Work out the finished part from the listing and answer in its coordinate system (mm). Give positions to 0.01 mm unless a question says otherwise; leave off trailing zeros. Order: outer loops, then holes, each group sorted by start corner. A loop starts at its lowest first (then second) coordinate and runs counter-clockwise, first axis right, second up. Notation, with made-up numbers: (63.25, 10.25) - (74.25, 10.25) arc R29 cw to (74.25, 37.25) - close; hole circle Ø8 at (-38.5, -34.5). An arc over 180 degrees is marked (long way). Write each question's results on one line, items separated by ' | '.
from build123d import *

# Parameters (mm, degrees)
SKICA1_W                 = 67
SKICA1_H                 = 107
P_IDAT_VYSUNUT_M1_DEPTH  = 3.5
ZAOBLIT1_R               = 3
SKICA2_R                 = 1.25
SKICA2_R_2               = 3
SKICA2_R_3               = 5.2
SKICA2_W                 = 41
SKICA2_H                 = 38
SKICA2_W_2               = 5.5
SKICA2_H_2               = 9
SKICA2_W_3               = 12.8
SKICA2_H_3               = 12.8
SKICA2_W_4               = 22.5
SKICA2_H_4               = 3.2
ODEBRAT_VYSUNUT_M1_DEPTH = 4.5
ZAOBLIT2_R               = 3
SKICA3_W                 = 22
SKICA3_H                 = 3
ODEBRAT_VYSUNUT_M2_DEPTH = 2
ZKOSEN_1_SIZE            = 1.3
SKICA4_W                 = 20.5
SKICA4_H                 = 8.5
ODEBRAT_VYSUNUT_M3_DEPTH = 1.2
SKICA5_W                 = 18.5
SKICA5_H                 = 6.5
ODEBRAT_VYSUNUT_M4_DEPTH = 3.3


with BuildPart() as part:
    # Skica1 → Přidat vysunutím1 (new body)
    with BuildSketch(Plane.XY):
        with Locations((33.5, 53.5)):
            Rectangle(SKICA1_W, SKICA1_H)
    extrude(amount=P_IDAT_VYSUNUT_M1_DEPTH)

    # Zaoblit1
    zaoblit1_edges = [part.edges().sort_by_distance(p)[0] for p in [
        (0, 107, 1.75),
        (67, 107, 1.75),
        (67, 0, 1.75),
        (0, 0, 1.75),
    ]]
    fillet(zaoblit1_edges, radius=ZAOBLIT1_R)

    # Skica2 → Odebrat vysunutím1 (cut, through all)
    with BuildSketch(Plane.XY.offset(3.5)):
        with Locations((6.5, 100.5)):
            Circle(SKICA2_R)
        with Locations((60.5, 100.5)):
            Circle(SKICA2_R)
        with Locations((6.5, 6.5)):
            Circle(SKICA2_R)
        with Locations((60.5, 6.5)):
            Circle(SKICA2_R)
        with Locations((7.3, 75.5)):
            Circle(SKICA2_R_2)
        with Locations((12.5, 12.5)):
            Circle(SKICA2_R_3)
        with Locations((26.5, 12.5)):
            Circle(SKICA2_R_3)
        with Locations((40.5, 12.5)):
            Circle(SKICA2_R_3)
        with Locations((54.5, 12.5)):
            Circle(SKICA2_R_3)
        with Locations((7.3, 84.5)):
            Circle(SKICA2_R_2)
        with Locations((33, 80.5)):
            Rectangle(SKICA2_W, SKICA2_H)
        with Locations((59.75, 76.5)):
            Rectangle(SKICA2_W_2, SKICA2_H_2)
        with Locations((54.5, 53.5)):
            Rectangle(SKICA2_W_3, SKICA2_H_3)
        with Locations((40.5, 53.5)):
            Rectangle(SKICA2_W_3, SKICA2_H_3)
        with Locations((26.5, 53.5)):
            Rectangle(SKICA2_W_3, SKICA2_H_3)
        with Locations((12.5, 53.5)):
            Rectangle(SKICA2_W_3, SKICA2_H_3)
        with Locations((50.65, 39.7)):
            Rectangle(SKICA2_W_4, SKICA2_H_4)
    extrude(amount=-ODEBRAT_VYSUNUT_M1_DEPTH, mode=Mode.SUBTRACT)

    # Zaoblit2
    zaoblit2_edges = [part.edges().sort_by_distance(p)[0] for p in [
        (6.1, 47.1, 1.75),
        (6.1, 59.9, 1.75),
        (18.9, 59.9, 1.75),
        (18.9, 47.1, 1.75),
        (20.1, 47.1, 1.75),
        (20.1, 59.9, 1.75),
        (32.9, 59.9, 1.75),
        (32.9, 47.1, 1.75),
        (34.1, 47.1, 1.75),
        (34.1, 59.9, 1.75),
        (46.9, 59.9, 1.75),
        (46.9, 47.1, 1.75),
        (48.1, 47.1, 1.75),
        (48.1, 59.9, 1.75),
        (60.9, 59.9, 1.75),
        (60.9, 47.1, 1.75),
    ]]
    fillet(zaoblit2_edges, radius=ZAOBLIT2_R)

    # Skica3 → Odebrat vysunutím2 (cut)
    with BuildSketch(Plane(origin=(0, 0, 0), x_dir=(-1, 0, 0), z_dir=(0, 0, -1))):
        with Locations((-33, 101)):
            Rectangle(SKICA3_W, SKICA3_H)
    extrude(amount=-ODEBRAT_VYSUNUT_M2_DEPTH, mode=Mode.SUBTRACT)

    # Zkosení1
    zkosen_1_edges = [part.edges().sort_by_distance(p)[0] for p in [
        (5.25, 6.5, 3.5),
        (59.25, 6.5, 3.5),
        (5.25, 100.5, 3.5),
        (59.25, 100.5, 3.5),
    ]]
    chamfer(zkosen_1_edges, length=ZKOSEN_1_SIZE)

    # Skica4 → Odebrat vysunutím3 (cut)
    with BuildSketch(Plane.XY.offset(3.5)):
        with Locations((16.35, 37.05)):
            Rectangle(SKICA4_W, SKICA4_H)
    extrude(amount=-ODEBRAT_VYSUNUT_M3_DEPTH, mode=Mode.SUBTRACT)

    # Skica5 → Odebrat vysunutím4 (cut, through all)
    with BuildSketch(Plane.XY.offset(2.3)):
        with Locations((16.35, 37.05)):
            Rectangle(SKICA5_W, SKICA5_H)
    extrude(amount=-ODEBRAT_VYSUNUT_M4_DEPTH, mode=Mode.SUBTRACT)


solid = part.part
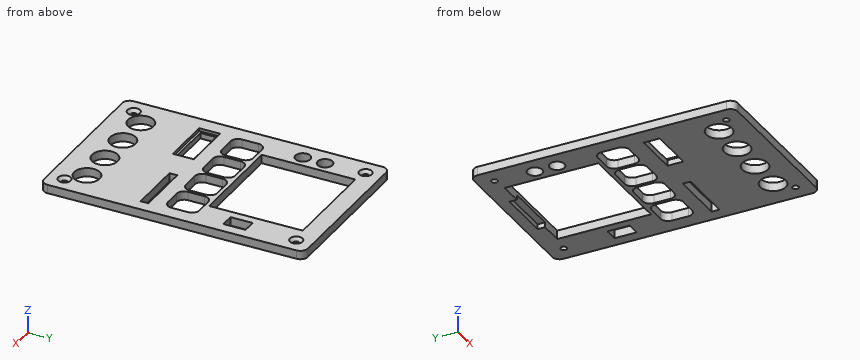
1. A cutting plane is placed at C-C, the plane z = 2.9. State how many separate pieces and enclosed holes the cut face has, then the cut area to 3 significant figures.
Answer list:
separate pieces: 1 | enclosed holes: 18 | area: 4,240 mm^2
2. A cutting plane is placed at A-A, the plane y = 12.5. Write down the section's boundary in (x, z), then the cut area to 3 significant figures.
Answer list:
outline: (0, 0) - (7.3, 0) - (7.3, 3.5) - (0, 3.5) - close; (17.7, 0) - (21.3, 0) - (21.3, 3.5) - (17.7, 3.5) - close; (31.7, 0) - (35.3, 0) - (35.3, 3.5) - (31.7, 3.5) - close; (45.7, 0) - (49.3, 0) - (49.3, 3.5) - (45.7, 3.5) - close; (59.7, 0) - (67, 0) - (67, 3.5) - (59.7, 3.5) - close | area: 88.9 mm^2
3. Given P1, Ø1.5, axis at x = 37, y = 101, coming from the -Z side, flat-ended and moving along its own axis, determine where the tip first touches the part or whether it passes through.
Answer list:
P1: z = 2
4. Straight lines are drawn through the part: line 1 (X direction, y = 53, z = 1.4); line 2 (Y direction, x = 54.5, z = 1.95); line 3 (X direction, y = 100.5, z = 0.95). For each, find the intervals that lie inside material, in ascending order. Write a range as [from, to].
Answer list:
line 1: [0, 6.1], [18.9, 20.1], [32.9, 34.1], [46.9, 48.1], [60.9, 67] | line 2: [0, 7.3], [17.7, 38.1], [41.3, 47.1], [59.9, 107] | line 3: [0, 5.25], [7.75, 22], [44, 59.25], [61.75, 67]
5. A cutting plane is placed at B-B, the plane y = 84.5. Write down the section's boundary in (x, z), then the cut area to 3 significant figures.
Answer list:
outline: (0, 0) - (4.3, 0) - (4.3, 3.5) - (0, 3.5) - close; (10.3, 0) - (12.5, 0) - (12.5, 3.5) - (10.3, 3.5) - close; (53.5, 0) - (67, 0) - (67, 3.5) - (53.5, 3.5) - close | area: 70.0 mm^2
